```python
from build123d import *

# Parameters (mm, degrees)
SKETCH1_R           = 50
BOSS_EXTRUDE1_DEPTH = 70
SKETCH2_W           = 50
SKETCH2_H           = 5
BOSS_EXTRUDE2_DEPTH = 150
SKETCH4_W           = 5
SKETCH4_H           = 50
BOSS_EXTRUDE3_DEPTH = 150


with BuildPart() as part:
    # Sketch1 → Boss-Extrude1 (new body)
    with BuildSketch(Plane.XY):
        Circle(SKETCH1_R)
    extrude(amount=BOSS_EXTRUDE1_DEPTH)

    # Sketch2 → Boss-Extrude2 (add)
    with BuildSketch(Plane(origin=(0, 0, 0), x_dir=(1, 0, 0), z_dir=(0, 1, 0))):
        with Locations((5, -67.5)):
            Rectangle(SKETCH2_W, SKETCH2_H)
    extrude(amount=BOSS_EXTRUDE2_DEPTH)

    # Sketch4 → Boss-Extrude3 (add)
    with BuildSketch(Plane(origin=(0, 0, 0), x_dir=(0, 0, -1), z_dir=(1, 0, 0))):
        with Locations((-2.5, 5)):
            Rectangle(SKETCH4_W, SKETCH4_H)
    extrude(amount=BOSS_EXTRUDE3_DEPTH)


solid = part.part
```
Geometry: final body of the model. Coordinates: model frame, mm. A direction names the side the tool comes from. Round coordinates to 2 decimals unless told otherwise and drop trailing zeros. Order: outer loops, then holes, each group sorted by start corner. A loop starts at its lowest first (then second) coordinate and runs counter-clockwise, first axis right, second up. Notation, with made-up numbers: M 4,0 L 13,0 A23 cw 13,12 Z; hole C -6,47.5 d6. An arc over 180 degrees is marked long. One line per item, written item: value.
(1) Cut plane D-D (y = 91.5). Return the cut outline in (x, z), and give its area (3 significant figures).
Result sheet:
outline: M -20,65 L 30,65 L 30,70 L -20,70 Z
area: 250 mm2
(2) Reachability of faces 1 (the cylindrical face through (-40, -30, 35)), 2 (the flat face through (97, -20, 3)), 3 (the flat face through (-20, 97, 68)), 4 (the flat face through (94, 30, 3)) from +Z, -Z, +X, -X, +Y, -Y: full face, straight path, thin tool, end or side. Return the list, or none.
Result sheet:
face 1: none
face 2: +Z, -Z, +X, -Y
face 3: +Z, -Z, -X, +Y
face 4: +Z, -Z, +X, +Y
(3) Cut plane C-C (z = 40). Return the cut outline in (x, y), and give its area (3 significant figures).
Result sheet:
outline: C 0,0 d100
area: 7,850 mm2
(4) Cut plane B-B (x = 0). Return the cut outline in (y, z).
Result sheet:
outline: M -50,0 L 50,0 L 50,65 L 150,65 L 150,70 L -50,70 Z
(5) Line query: probe 1 along X at (y, z) = (109, 66); probe 2 along Z at (x, y) = (10, 121); probe 3 along X at (y, z) = (-2, 10.5). Output: solid intervals per line, ascending. Write a range as [from, to].
Result sheet:
probe 1: [-20, 30]
probe 2: [65, 70]
probe 3: [-49.96, 49.96]
(6) Cut plane A-A (y = 0). Return the cut outline in (x, z), and give its area (3 significant figures).
Result sheet:
outline: M -50,0 L 150,0 L 150,5 L 50,5 L 50,70 L -50,70 Z
area: 7,500 mm2
(7) Pin query (flat end, axial travel): P1, Ø8, axis at x = 49, z = 42, coming from the +Y side; P2, Ø4, axis at y = 19, z = 56, coming from the -X side; P3, Ø5.5, axis at y = 104.5, z = 68, coming from the -X side. Return the tip coordinate at first contact, or that it passes through.
Result sheet:
P1: y = 21.79
P2: x = -47.02
P3: x = -20
